Work out the finished part from the listing and answer in its coordinate system (mm). A direction names the side the tool comes from. Coordinates: 2 decimals unless noted, no trailing zeros. Write each loop counter-clockwise with the first axis right and the second up, starting at its lowest first coordinate (ties: lowest second). Pieces come first, ordered by that corner, then holes. Notation, with made-up numbers: (16, 69) - (64, 69) arc R31 ccw to (64, 107) - close; hole circle Ø5 at (55.5, 86). An arc over 180 degrees is marked (long way). Answer as a JSON object with one key per item and string values. Group by question number.
from build123d import *

# Parameters (mm, degrees)
F1_DEPTH    = 112
F2_R        = 25
F3_DEPTH    = 185
F2_R_2      = 31.5
F5_DEPTH    = 184
F6_DEPTH    = 95
F7_W        = 47
F7_H        = 100
F8_DEPTH    = 159
F9_R        = 5.5
F10_DEPTH   = 157.2
F9_R_2      = 1.5
F11_DEPTH   = 154.4
F12_SIZE2   = 32
F12_SIZE    = 20
F12_2_SIZE2 = 32
F12_2_SIZE  = 20
F13_SIZE    = 2.5


with BuildPart() as f1:
    # F0 (on Front) → F1 (new body)
    with BuildSketch(Plane.XZ):
        with BuildLine():
            ThreePointArc((-59.7957043946, -22.8214863997), (-55.1094128936, -34.1351948987), (-43.7957043946, -38.8214863997))
            Line((-43.7957043946, -38.8214863997), (19.2042956054, -38.8214863997))
            ThreePointArc((19.2042956054, -38.8214863997), (30.5180041044, -34.1351948987), (35.2042956054, -22.8214863997))
            Line((35.2042956054, -22.8214863997), (35.2042956054, 103.1785136003))
            Line((35.2042956054, 103.1785136003), (29.2042956054, 103.1785136003))
            Line((29.2042956054, 103.1785136003), (29.2042956054, 87.1785136003))
            Line((29.2042956054, 87.1785136003), (29.2042956054, -23.8214863997))
            ThreePointArc((29.2042956054, -23.8214863997), (26.5682566361, -30.1854474304), (20.2042956054, -32.8214863997))
            Line((20.2042956054, -32.8214863997), (-44.7957043946, -32.8214863997))
            ThreePointArc((-44.7957043946, -32.8214863997), (-51.1596654253, -30.1854474304), (-53.7957043946, -23.8214863997))
            Line((-53.7957043946, -23.8214863997), (-53.7957043946, 86.1785136003))
            Line((-53.7957043946, 86.1785136003), (-59.7957043946, 86.1785136003))
            Line((-59.7957043946, 86.1785136003), (-59.7957043946, -22.8214863997))
        make_face()
    extrude(amount=F1_DEPTH)

    # F2 (on face) → F3 (cut)
    with BuildSketch(Plane.YZ.offset(35.2042956054)):
        with Locations((-56, 47.1785136003)):
            Circle(F2_R)
    extrude(amount=-F3_DEPTH, mode=Mode.SUBTRACT)

    # F2 (on face) → F5 (cut)
    with BuildSketch(Plane.YZ.offset(35.2042956054)):
        with Locations((-56, 47.1785136003)):
            Circle(F2_R_2)
        with Locations((-56, 47.1785136003)):
            Circle(F2_R, mode=Mode.SUBTRACT)
    extrude(amount=-F5_DEPTH, mode=Mode.SUBTRACT)

    # F2 (on face) → F6 (join)
    with BuildSketch(Plane.YZ.offset(35.2042956054)):
        with Locations((-56, 47.1785136003)):
            Circle(F2_R_2)
        with Locations((-56, 47.1785136003)):
            Circle(F2_R, mode=Mode.SUBTRACT)
    extrude(amount=-F6_DEPTH)

    # F7 (on offset) → F8 (cut)
    with BuildSketch(Plane.XZ.offset(137)):
        with Locations((-11.2957043946, 29.1785136003)):
            Rectangle(F7_W, F7_H)
    extrude(amount=-F8_DEPTH, mode=Mode.SUBTRACT)

    # F9 (on face) → F10 (cut)
    with BuildSketch(Plane.YZ.offset(35.2042956054)):
        with Locations((-83, 92.1785136003)):
            Circle(F9_R)
        with Locations((-29, 92.1785136003)):
            Circle(F9_R)
        with Locations((-95, 7.1785136003)):
            Circle(F9_R)
        with Locations((-17, 7.1785136003)):
            Circle(F9_R)
    extrude(amount=-F10_DEPTH, mode=Mode.SUBTRACT)

    # F9 (on face) → F11 (cut)
    with BuildSketch(Plane.YZ.offset(35.2042956054)):
        with Locations((-31.751288694, 33.2468845546)):
            Circle(F9_R_2)
        with Locations((-80.248711306, 33.2468845546)):
            Circle(F9_R_2)
        with BuildLine():
            ThreePointArc((-56, 73.7468845546), (-54.9393398282, 74.1862243828), (-54.5, 75.2468845546))
            ThreePointArc((-54.5, 75.2468845546), (-57.0606601718, 76.3075447264), (-56, 73.7468845546))
        make_face()
    extrude(amount=-F11_DEPTH, mode=Mode.SUBTRACT)

    # F12
    f12_edges = [f1.edges().sort_by_distance(p)[0] for p in [
        (-56.795704, 0, 86.178514),
        (-56.795704, -112, 86.178514),
    ]]
    f12_side = f1.faces().sort_by_distance((-56.795704, -56, 86.178514))[0]
    chamfer(f12_edges, length=F12_SIZE, length2=F12_SIZE2, reference=f12_side)

    # F12#2
    f12_2_edges = [f1.edges().sort_by_distance(p)[0] for p in [
        (32.204296, 0, 103.178514),
        (32.204296, -112, 103.178514),
    ]]
    f12_2_side = f1.faces().sort_by_distance((32.204296, -56, 103.178514))[0]
    chamfer(f12_2_edges, length=F12_2_SIZE, length2=F12_2_SIZE2, reference=f12_2_side)

    # F13
    f13_edges = [f1.edges().sort_by_distance(p)[0] for p in [
        (-59.795704, -22.5, 7.178514),
        (-59.795704, -100.5, 7.178514),
    ]]
    chamfer(f13_edges, length=F13_SIZE)


solid = f1.part
Q1. Flat-ended cylindrical pins translate along their axes: pin 1 Ø19.5 at (x, y) = (2, -35) entering from +Z; pin 2 Ø12 at (x, z) = (11.5, 47.5) entering from +Y; pin 3 Ø1.8 at (x, y) = (-57.5, -63.5) entering from +Z. Find the tip coordinate at first contact, or state that the pin passes through.
Q2. Consider L1, parallel to X at y = -22.5, z = -14; L2, parallel to X at y = -81.5, z = 53; L3, parallel to Z at x = 25.5, y = -70. Determine where each line is inside the solid, lowest interval first. Write a range as from..to.
Q3. A tool of negligible diameter and unlimited length cuts with its end or side. For faces 5 (the face through (-53.796, -43, 18)), 6 (the face through (-51.089, -55.216, -30.255)), 7 (the face through (-56.754, -102.14, 69.955)), 8 (the face through (-55.233, -55.216, -34.01)), from which of +Z, -Z, +X, -X, +Y, -Y can it reach the whole face along a straight path? Write none if from no direction.
Q4. For a pull along X with two mould halves and no side action, classify faces 1 (the face through (-57.42, -100.62, 7.43)), 2 (the face through (35.204, -43, 25)), 3 (the face through (-56.754, -9.86, 69.955)), 4 (the face through (26.638, -55.216, -30.115)) as +X half, -X half, draft (parallel to the pull), parting line (faces both ways), or undercut.
Q5. Section D-D on z = 59 is taken. Determine the outline of the cut face in (x, y), plus the area to 3 significant figures.
Q6. Section A-A on x = 23.5 is taken. Determine the outline of the cut face in (y, z).
Q7. Section C-C on z = -30 is taken. Determine the outline of the cut face in (x, y), plus the area to 3 significant figures.
Q8. Section B-B on y = -85 is taken. Determine the outline of the cut face in (x, z), plus the area to 3 significant figures.
Numbers:
{
 "1": {"pin 1": "stops at z = -32.82", "pin 2": "stops at y = -24.5", "pin 3": "stops at z = 86.18"},
 "2": {"L1": "x = -59.8..-53.8, 29.2..35.2", "L2": "x = -59.8..-34.8, 12.2..35.2", "L3": "z = -37.53..-31.1, 18.96..26.47, 67.89..75.4"},
 "3": {"face 5": "none", "face 6": "+Y, -Y", "face 7": "+Z, -X, -Y", "face 8": "-Z, -X, +Y, -Y"},
 "4": {"face 1": "-X half", "face 2": "+X half", "face 3": "draft", "face 4": "undercut"},
 "5": {"outline": "(-59.8, -108.99) - (-53.8, -108.99) - (-53.8, -85.2) - (-34.8, -85.2) - (-34.8, -78.03) - (-59.8, -78.03) - close; (-59.8, -33.97) - (-34.8, -33.97) - (-34.8, -26.8) - (-53.8, -26.8) - (-53.8, -3.01) - (-59.8, -3.01) - close; (12.2, -85.2) - (29.2, -85.2) - (29.2, -112) - (35.2, -112) - (35.2, -78.03) - (12.2, -78.03) - close; (12.2, -33.97) - (35.2, -33.97) - (35.2, 0) - (29.2, 0) - (29.2, -26.8) - (12.2, -26.8) - close", "area": "1,300 mm²"},
 "6": {"outline": "(-112, -38.23) - (0, -38.23) - (0, -32.2) - (-112, -32.2) - close; circle Ø63 at (-56, 47.18); hole circle Ø3 at (-80.25, 33.25); hole circle Ø50 at (-56, 47.18); hole circle Ø3 at (-56, 75.25); hole circle Ø3 at (-31.75, 33.25)"},
 "7": {"outline": "(-58.09, -112) - (-51.34, -112) - (-51.34, 0) - (-58.09, 0) - close; (26.75, -112) - (33.5, -112) - (33.5, 0) - (26.75, 0) - close", "area": "1,510 mm²"},
 "8": {"outline": "(-59.8, -22.82) arc R16 ccw to (-43.8, -38.82) - (19.2, -38.82) arc R16 ccw to (35.2, -22.82) - (35.2, 87.06) - (29.2, 87.06) - (29.2, 59.48) - (12.2, 59.48) - (12.2, 34.88) - (29.2, 34.88) - (29.2, -23.82) arc R9 cw to (20.2, -32.82) - (-44.8, -32.82) arc R9 cw to (-53.8, -23.82) - (-53.8, 34.88) - (-34.8, 34.88) - (-34.8, 59.48) - (-53.8, 59.48) - (-53.8, 86.18) - (-59.8, 86.18) - close; (29.2, 97.3) - (35.2, 97.3) - (35.2, 103.18) - (29.2, 103.18) - close", "area": "2,850 mm²"}
}
